```python
from build123d import *

# Parameters (mm, degrees)
SKETCH1_W                       = 20
SKETCH1_H                       = 20
BOSS_EXTRUDE1_DEPTH             = 110
FILLET1_R                       = 10
SKETCH2_R                       = 6.5
CUT_EXTRUDE1_DEPTH              = 20
F_2_0MM_DOWEL_HOLE1_D           = 2
F_2_0MM_DOWEL_HOLE1_CSINK_D     = 2.05
F_2_0MM_DOWEL_HOLE1_CSINK_ANGLE = 90


with BuildPart() as part:
    # Sketch1 → Boss-Extrude1 (new body)
    with BuildSketch(Plane(origin=(0, 0, 0), x_dir=(0, 1, 0), z_dir=(0, 0, 1))):
        Rectangle(SKETCH1_W, SKETCH1_H)
    extrude(amount=-BOSS_EXTRUDE1_DEPTH)

    # Fillet1
    fillet1_edges = [part.edges().sort_by_distance(p)[0] for p in [
        (0, -10, -110),
        (0, 10, -110),
    ]]
    fillet(fillet1_edges, radius=FILLET1_R - 0.0001)  # a hair under: the kernel refuses the full size

    # Sketch2 → Cut-Extrude1 (cut)
    with BuildSketch(Plane.YZ.offset(10)):
        with Locations((0, -100)):
            Circle(SKETCH2_R)
    extrude(amount=-CUT_EXTRUDE1_DEPTH, mode=Mode.SUBTRACT)

    # Ø2.0mm Dowel Hole1 (through all)
    with Locations(Plane.XZ.offset(10)):
        with Locations((0, -5)):
            f_2_0mm_dowel_hole1 = CounterSinkHole(F_2_0MM_DOWEL_HOLE1_D / 2, F_2_0MM_DOWEL_HOLE1_CSINK_D / 2, counter_sink_angle=F_2_0MM_DOWEL_HOLE1_CSINK_ANGLE)

    # Mirror1: Ø2.0mm Dowel Hole1 across plane
    add(f_2_0mm_dowel_hole1.mirror(Plane.ZX), mode=Mode.SUBTRACT)


solid = part.part
```
Geometry check sheet. Reference: the model listing, model coordinates, mm. Coordinates: 2 decimals unless noted, no trailing zeros. Loops run counter-clockwise (first coordinate to the right, second up) from the corner with the lowest first, then second, coordinate; pieces in that order, holes last. Notation, with made-up numbers: (1, -3.75) -> (6, -3.75) arc R21 ccw to (6, 22.25) -> close; hole circle Ø7 at (-37, 50). An arc over 180 degrees is marked (long way). Put each result on its own line as item: value.
1) Gauge pin test, flat ends, axial feed: pin 1 Ø2 at (x, y) = (7.5, 5.5) entering from +Z; pin 2 Ø1 at (x, y) = (-6.5, -7.5) entering from -Z; pin 3 Ø6 at (x, y) = (-1, -5.5) entering from -Z. Record the tip position at first contact, or that the pin passes through.
Result set:
pin 1: stops at z = 0
pin 2: stops at z = -107.14
pin 3: stops at z = -109.68
2) Cross-section at A-A on x = 0. Count the separate pieces of the cut face and the enclosed holes in it, plus the area to 3 significant figures.
Result set:
separate pieces: 2
enclosed holes: 1
area: 1,980 mm^2
3) Release check for a two-part mould opening along X. For faces 1 (the flat face through (-10, 0, -54)), 2 (the flat face through (0, 0, 0)), 3 (the cylindrical face through (0, 0, -4)) record: released by +X, released by -X, zero draft, split by the parting line, or undercut.
Result set:
face 1: released by -X
face 2: zero draft
face 3: undercut
4) Cross-section at B-B on y = -1.5. Record the boundary of the cut face in (x, z), plus the area to 3 significant figures.
Result set:
outline: (-10, -109.89) -> (10, -109.89) -> (10, -106.32) -> (-10, -106.32) -> close; (-10, -93.68) -> (10, -93.68) -> (10, 0) -> (-10, 0) -> close; hole circle Ø2 at (0, -5)
area: 1,940 mm^2
5) Cross-section at C-C on z = -5. Record the boundary of the cut face in (x, y) (3 decimals), plus the area to 3 significant figures.
Result set:
outline: (-10, -10) -> (-1.025, -10) -> (-1, -9.975) -> (-1, 9.975) -> (-1.025, 10) -> (-10, 10) -> close; (1, -9.975) -> (1.025, -10) -> (10, -10) -> (10, 10) -> (1.025, 10) -> (1, 9.975) -> close
area: 360 mm^2
6) Thickness scan on line 1 (Z direction, x = 4.25, y = 0); line 2 (Z direction, x = 0, y = -2.5); line 3 (X direction, y = -0.25, z = -5). Record the ranges inside material, lowest first.
Result set:
line 1: z = -110 to -106.5, -93.5 to 0
line 2: z = -109.68 to -106, -94 to -6, -4 to 0
line 3: x = -10 to -1, 1 to 10
